Can you work these out from the model? Positions are in its coordinate system, mm. Give positions to 0.01 mm unless a question says otherwise; leave off trailing zeros. Loops run counter-clockwise (first coordinate to the right, second up) from the corner with the lowest first, then second, coordinate; pieces in that order, holes last. Notation, with made-up numbers: (61.5, -29) - (74.5, -29) arc R8 cw to (74.5, -18) - close; hole circle Ø2 at (59.25, -30). An arc over 180 degrees is marked (long way). Write item = value, one per line.
from build123d import *

# Parameters (mm, degrees)
SKETCH_1_R      = 7.55
SKETCH_1_R_2    = 6.1
SKETCH_1_R_3    = 3.05
EXTRUDE_1_DEPTH = 2


with BuildPart() as part:
    # 草图1 → 凸台-拉伸1 (new body)
    with BuildSketch(Plane(origin=(0, 0, 0), x_dir=(0, 0, -1), z_dir=(1, 0, 0))):
        with BuildLine():
            Line((19.426316451, -58.647367097), (-125.573683549, -58.647367097))
            ThreePointArc((-125.573683549, -58.647367097), (-150.573683549, -33.647367097), (-125.573683549, -8.647367097))
            Line((-125.573683549, -8.647367097), (4.992559722, -8.647367097))
            Line((4.992559722, -8.647367097), (19.426316451, -8.647367097))
            ThreePointArc((19.426316451, -8.647367097), (44.426316451, -33.647367097), (19.426316451, -58.647367097))
        make_face()
        with Locations((19.426316451, -33.647367097)):
            Circle(SKETCH_1_R, mode=Mode.SUBTRACT)
        with Locations((-125.573683549, -33.647367097)):
            Circle(SKETCH_1_R_2, mode=Mode.SUBTRACT)
        with Locations((-56.921571535, -43.647367097)):
            Circle(SKETCH_1_R_3, mode=Mode.SUBTRACT)
        with Locations((-15.573683549, -15.647367097)):
            Circle(SKETCH_1_R_3, mode=Mode.SUBTRACT)
        with Locations((-55.573683549, -15.647367097)):
            Circle(SKETCH_1_R_3, mode=Mode.SUBTRACT)
    extrude(amount=EXTRUDE_1_DEPTH)


solid = part.part
Q1. Imagine slicing it at B-B, the plane x = 0.95. Write out the boundary of the cut face in (y, z), then the cut area to 3 significant figures.
Output:
outline = (-58.65, -19.43) arc R25 ccw to (-8.65, -19.43) - (-8.65, 125.57) arc R25 ccw to (-58.65, 125.57) - close; hole circle Ø6.1 at (-43.65, 56.92); hole circle Ø15.1 at (-33.65, -19.43); hole circle Ø12.2 at (-33.65, 125.57); hole circle Ø6.1 at (-15.65, 15.57); hole circle Ø6.1 at (-15.65, 55.57)
area = 8,830 mm2
Q2. Imagine slicing it at C-C, the plane y = -52. Write out the boundary of the cut face in (x, z).
Output:
outline = (0, -36.4) - (2, -36.4) - (2, 142.55) - (0, 142.55) - close
Q3. Imagine slicing it at A-A, the plane z = -17.5. Write out the boundary of the cut face in (x, y), then the cut area to 3 significant figures.
Output:
outline = (0, -58.65) - (2, -58.65) - (2, -40.95) - (0, -40.95) - close; (0, -26.35) - (2, -26.35) - (2, -8.65) - (0, -8.65) - close
area = 70.8 mm2
Q4. We'd pull the mould along Y, two halves only. Please class faces 1 (the cylindrical face through (0.99, -33.1, -44.42)), 2 (the cylindrical face through (0.986, -27.281, -23.485)), 3 (the cylindrical face through (0.986, -31.815, 119.755)), 4 (the flat face through (2, -33, 52)): released by +Y, released by -Y, zero draft, split by the parting line, or undercut.
Output:
face_1 = split by the parting line
face_2 = undercut
face_3 = undercut
face_4 = zero draft
Q5. For pin 1 (5 mm diameter, centred on y = -43.65, z = 56.92, fed in from +X); pin 2 (1 mm diameter, centred on x = 1, y = -31.5, fed in from -Z), each with a flat end and sliding along its axis, tell me the tip position at first contact or that it passes through.
Output:
pin_1 = through
pin_2 = -44.37
Q6. I need wall thicknesses on L1, parallel to Z at x = 1.4, y = -31.5; L2, parallel to Z at x = 1.15, y = -14.5; L3, parallel to Y at x = 1.3, z = 58. Which ranges of each line are inside material? Lowest first, please.
Output:
L1 = -44.33 to -26.66, -12.19 to 119.86, 131.28 to 150.48
L2 = -35.5 to 12.75, 18.4 to 52.75, 58.4 to 141.65
L3 = -58.65 to -46.5, -40.79 to -17.5, -13.8 to -8.65
